```python
from build123d import *

# Parameters (mm, degrees)
F1_DEPTH = 12.7
F3_DEPTH = 12.701
F5_DEPTH = 12.701
F6_W     = 152.4
F6_H     = 5.08
F7_DEPTH = 12.701
F8_R     = 1.27


with BuildPart() as f1:
    # F0 (on Top) → F1 (new body)
    with BuildSketch(Plane.XY):
        with BuildLine():
            ThreePointArc((-177.8, 609.6), (-45.357143, 317.5), (0, 0))
            Line((0, 0), (177.8, 0))
            ThreePointArc((177.8, 0), (132.442857, 317.5), (0, 609.6))
            Line((0, 609.6), (-177.8, 609.6))
        make_face()
    extrude(amount=F1_DEPTH)

    # F2 (on face) → F3 (cut, through all)
    with BuildSketch(Plane.XY.offset(12.7)):
        with BuildLine():
            Line((44.6749, 25.4), (49.7549, 25.4))
            ThreePointArc((49.7549, 25.4), (1.163489, 314.204707), (-112.290582, 584.2))
            Line((-112.290582, 584.2), (-117.370582, 584.2))
            ThreePointArc((-117.370582, 584.2), (-3.916511, 314.204707), (44.6749, 25.4))
        make_face()
    extrude(amount=-F3_DEPTH, mode=Mode.SUBTRACT)

    # F4 (on face) → F5 (cut, through all)
    with BuildSketch(Plane.XY.offset(12.7)):
        with BuildLine():
            ThreePointArc((-36.090582, 584.2), (77.363489, 314.204707), (125.9549, 25.4))
            Line((125.9549, 25.4), (131.0349, 25.4))
            ThreePointArc((131.0349, 25.4), (82.443489, 314.204707), (-31.010582, 584.2))
            Line((-31.010582, 584.2), (-36.090582, 584.2))
        make_face()
    extrude(amount=-F5_DEPTH, mode=Mode.SUBTRACT)

    # F6 (on face) → F7 (cut, through all)
    with BuildSketch(Plane.XY.offset(12.7)):
        with Locations((88.9, 10.16)):
            Rectangle(F6_W, F6_H)
    extrude(amount=-F7_DEPTH, mode=Mode.SUBTRACT)

    # F8
    f8_edges = [f1.edges().sort_by_distance(p)[0] for p in [
        (-114.830582, 584.2, 12.7),
        (1.163489, 314.204707, 12.7),
        (-3.916511, 314.204707, 12.7),
        (47.2149, 25.4, 12.7),
        (88.9, 12.7, 12.7),
        (12.7, 10.16, 12.7),
        (88.9, 7.62, 12.7),
        (165.1, 10.16, 12.7),
        (82.443489, 314.204707, 12.7),
        (77.363489, 314.204707, 12.7),
        (128.4949, 25.4, 12.7),
        (-33.550582, 584.2, 12.7),
        (-114.830582, 584.2, 0),
        (1.163489, 314.204707, 0),
        (-3.916511, 314.204707, 0),
        (47.2149, 25.4, 0),
        (128.4949, 25.4, 0),
        (82.443489, 314.204707, 0),
        (77.363489, 314.204707, 0),
        (-33.550582, 584.2, 0),
        (12.7, 10.16, 0),
        (88.9, 12.7, 0),
        (88.9, 7.62, 0),
        (165.1, 10.16, 0),
    ]]
    fillet(f8_edges, radius=F8_R)


solid = f1.part
```
Verification items for the finished model (mm, model axes). A direction names the side the tool comes from. Give positions to 0.01 mm unless a question says otherwise; leave off trailing zeros. Loops run counter-clockwise (first coordinate to the right, second up) from the corner with the lowest first, then second, coordinate; pieces in that order, holes last. Notation, with made-up numbers: M 60,64 L 78,64 A13 cw 78,78 Z; hole C 9.25,24.25 d2. An arc over 180 degrees is marked long. One line per question, with ' | ' between items.
Item 1: Depth check by flat-ended pin: P1, Ø4, axis at y = 330, z = 2, coming from the +X side; P2, Ø6, axis at y = 450, z = 2.5, coming from the +X side; P3, Ø3, axis at y = 280, z = 9, coming from the +X side. Enter the tip coordinate at first touch or a pass-through.
Completed:
P1: stops at x = 129.33 | P2: stops at x = 85.98 | P3: stops at x = 143.07
Item 2: Section check A-A, the plane z = 5. Record the cut outline in (x, y).
Completed:
outline: M -177.8,609.6 A1133.93 cw 0,0 L 177.8,0 A1133.93 ccw 0,609.6 Z; hole M -117.37,584.2 A1270 cw 44.67,25.4 L 49.75,25.4 A1270 ccw -112.29,584.2 Z; hole M -36.09,584.2 A1270 cw 125.95,25.4 L 131.03,25.4 A1270 ccw -31.01,584.2 Z; hole M 12.7,7.62 L 165.1,7.62 L 165.1,12.7 L 12.7,12.7 Z
Item 3: Tool access check on faces 5 (the face through (83.58, 310.26, 6.42)), 6 (the face through (133.696, 313.172, 6.261)). Record the directions out of +Z, -Z, +X, -X, +Y, -Y that give a thin tool (end or side, any length) a straight path to the whole face; none if there is none.
Completed:
face 5: +Z, -Z | face 6: +Z, -Z, +X, +Y
Item 4: Draft check along Y on faces 1 (the face through (37, 309, 12.7)), 2 (the face through (-5.067, 318.149, 6.421)), 3 (the face through (2.3, 310.26, 6.42)), 4 (the face through (-88, 609.6, 6)). Enter one of: +Y half, -Y half, draft (parallel to the pull), parting line (faces both ways), or undercut.
Completed:
face 1: draft | face 2: undercut | face 3: undercut | face 4: +Y half
Item 5: Section check B-B, the plane x = 73. State how many separate pieces and enclosed holes the cut face has, plus the area to 3 significant figures.
Completed:
separate pieces: 3 | enclosed holes: 0 | area: 5,770 mm^2
Item 6: Thickness scan on line 1 (X direction, y = 385, z = 2.5); line 2 (X direction, y = 365.5, z = 4.25); line 3 (Y direction, x = -91, z = 1.25). Record the ranges inside material, lowest first. Write a range as [from, to].
Completed:
line 1: x = [-67.36, -26.71], [-21.63, 54.57], [59.65, 110.44] | line 2: x = [-60.52, -19.98], [-14.9, 61.3], [66.38, 117.28] | line 3: y = [445.08, 534.92], [544.83, 609.6]
Item 7: Section check D-D, the plane x = -129. Record the cut outline in (y, z), plus the area to 3 significant figures.
Completed:
outline: M 525.27,0 L 609.6,0 L 609.6,12.7 L 525.27,12.7 Z | area: 1,070 mm^2
